Could you check a few things on this drawing? It's one solid part, dimensions in mm from its lowest x, y, z. Coordinates: 2 decimals unless noted, no trailing zeros. Loops run counter-clockwise (first coordinate to the right, second up) from the corner with the lowest first, then second, coordinate; pieces in that order, holes last.
1) Will these pins go through, and if not, where does the flat tip stop? P1, Ø4, axis at y = 246.5, z = 3, coming from the +X side; P2, Ø4, axis at y = 227.5, z = 1.5, coming from the -X side.
2) Imagine slicing it at A-A on z = 4. Please give me the cut outline in (x, y), plus the area to 3 significant figures.
3) If I drill on line 1 along Y through (x, z) = (1.05, 4); line 2 along Y through (x, z) = (3, 4.5); line 3 along Y through (x, z) = (5, 4.5), over which ranges is the centre line in solid material (lowest first)?
4) Imagine slicing it at B-B on y = 218. Please give me the cut outline in (x, z), plus the area to 3 significant figures.
5) Imagine slicing it at C-C on x = 6.25. Please give me the cut outline in (y, z).
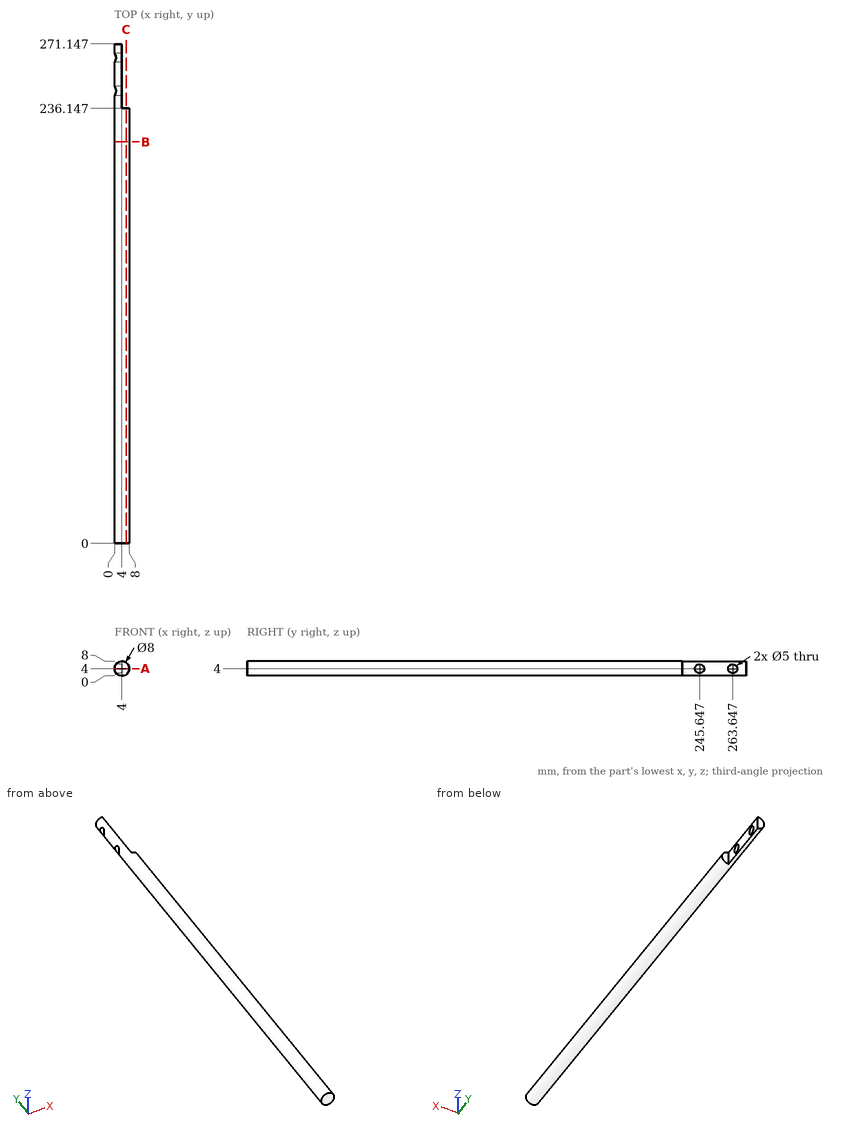
Filled in:
1. P1: stops at x = 4
1. P2: stops at x = 0.03
2. outline: (0, 0) - (8, 0) - (8, 236.15) - (4, 236.15) - (4, 243.15) - (0, 243.15) - close; (0, 248.15) - (4, 248.15) - (4, 261.15) - (0, 261.15) - close; (0, 266.15) - (4, 266.15) - (4, 271.15) - (0, 271.15) - close
2. area: 1,990 mm2
3. line 1: y = 0 to 243.15, 248.15 to 261.15, 266.15 to 271.15
3. line 2: y = 0 to 243.2, 248.1 to 261.2, 266.1 to 271.15
3. line 3: y = 0 to 236.15
4. outline: circle Ø8 at (4, 4)
4. area: 50.3 mm2
5. outline: (0, 0.69) - (236.15, 0.69) - (236.15, 7.31) - (0, 7.31) - close
